Verification items for this drawing (mm, ordinates from the low corner). Give positions to 0.01 mm unless a question says otherwise; leave off trailing zeros. Order: outer loops, then holes, each group sorted by start corner. A loop starts at its lowest first (then second) coordinate and runs counter-clockwise, first axis right, second up.
(1) Sectioned sample at D-D on x = 57. Record the cut outline in (y, z).
(2) Sectioned sample at A-A on z = 25.5. Record the cut outline in (x, y), plus the area to 3 significant figures.
(3) Gauge pin test, flat end, axial feed: pin 1 (15 mm diameter, centred on x = 39.95, z = 25.5, fed in from -Y). Record the tip position at first contact, or that the pin passes through.
(4) Mould release check, pull along X, two halves, no side actions. Record for the marked faces 1, 2 and 3: pulls with the +X half, pulls with the -X half, needs draft (parallel to the pull), parting line crosses it, or undercut.
(5) Sectioned sample at B-B on y = 2.5. Record the cut outline in (x, z).
(6) Sectioned sample at C-C on z = 14.5. Record the cut outline in (x, y).
(7) Scan lines: L1, parallel to X at y = 3.25, z = 25.5; L2, parallel to Z at x = 46.5, y = 3.75 (1 decimal); L3, parallel to X at y = 7.75, z = 19.5 (1 decimal). Record each from-to range of solid material in increasing order.
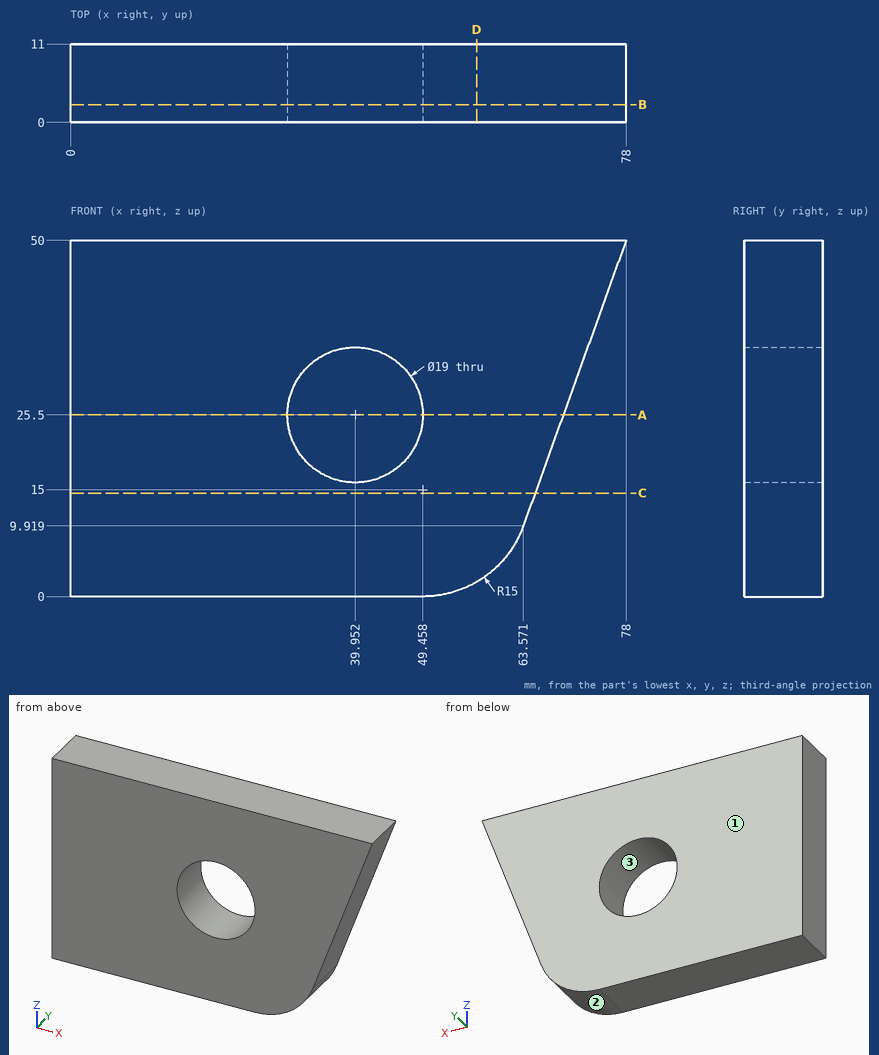
Ans:
1. outline: (0, 2.03) - (11, 2.03) - (11, 50) - (0, 50) - close
2. outline: (0, 0) - (30.45, 0) - (30.45, 11) - (0, 11) - close; (49.45, 0) - (69.18, 0) - (69.18, 11) - (49.45, 11) - close
2. area: 552 mm2
3. pin 1: passes through
4. face 1: needs draft
4. face 2: pulls with the +X half
4. face 3: undercut
5. outline: (0, 0) - (49.46, 0) arc R15 ccw to (63.57, 9.92) - (78, 50) - (0, 50) - close; hole circle Ø19 at (39.95, 25.5)
6. outline: (0, 0) - (65.22, 0) - (65.22, 11) - (0, 11) - close
7. L1: x = 0 to 30.45, 49.45 to 69.18
7. L2: z = 0 to 18.6, 32.4 to 50
7. L3: x = 0 to 32.6, 47.3 to 67
